Source: CAD feature listing. Evaluate the final solid. Frame: model axes, mm. Give positions to 0.01 mm unless a question says otherwise; leave off trailing zeros. Use a Markdown table: item, result. Add a question column.
```python
from build123d import *

# Parameters (mm, degrees)
SKETCH1_R           = 1.75
BOSS_EXTRUDE1_DEPTH = 5
CUT_EXTRUDE1_DEPTH  = 5
FILLET2_R           = 2


with BuildPart() as part:
    # Sketch1 → Boss-Extrude1 (new body)
    with BuildSketch(Plane(origin=(0, 0, 0), x_dir=(1, 0, 0), z_dir=(0, 1, 0))):
        with BuildLine():
            Line((-115, 97), (-115, -97))
            ThreePointArc((-115, -97), (-114.121320344, -99.121320344), (-112, -100))
            Line((-112, -100), (112, -100))
            ThreePointArc((112, -100), (114.121320344, -99.121320344), (115, -97))
            Line((115, -97), (115, 8.326847539))
            ThreePointArc((115, 8.326847539), (114.595001354, 9.832160786), (113.489354684, 10.931040816))
            Line((113.489354684, 10.931040816), (112.482257806, 11.50700592))
            Line((112.482257806, 11.50700592), (-41.694544071, 99.604753313))
            ThreePointArc((-41.694544071, 99.604753313), (-42.412938544, 99.899505125), (-43.182919083, 100))
            Line((-43.182919083, 100), (-112, 100))
            ThreePointArc((-112, 100), (-114.121320344, 99.121320344), (-115, 97))
        make_face()
        with Locations(Location((-107.357965586, 91.996726093, 0), (0, 0, 270))):
            Circle(SKETCH1_R, mode=Mode.SUBTRACT)
        with Locations(Location((107.171572875, 4.338256462, 0), (0, 0, 270))):
            Circle(SKETCH1_R, mode=Mode.SUBTRACT)
        with Locations(Location((107.171572875, -92.171572875, 0), (0, 0, 270))):
            Circle(SKETCH1_R, mode=Mode.SUBTRACT)
        with Locations(Location((-107.320588757, -92.030024345, 0), (0, 0, 270))):
            Circle(SKETCH1_R, mode=Mode.SUBTRACT)
    extrude(amount=BOSS_EXTRUDE1_DEPTH)

    # Sketch2 → Cut-Extrude1 (cut)
    with BuildSketch(Plane(origin=(0, 5, 0), x_dir=(1, 0, 0), z_dir=(0, 1, 0))):
        with BuildLine():
            ThreePointArc((83.411536631, -17.554766753), (65, -11.836576231), (46.588463369, -17.554766753))
            Line((46.588463369, -17.554766753), (83.411536631, -17.554766753))
        make_face()
        with BuildLine():
            ThreePointArc((42.258724115, -21.118385708), (39.509391878, -24.17525441), (37.167988383, -27.554766753))
            Line((37.167988383, -27.554766753), (92.832011617, -27.554766753))
            ThreePointArc((92.832011617, -27.554766753), (90.490608122, -24.17525441), (87.741275885, -21.118385708))
            Line((87.741275885, -21.118385708), (42.258724115, -21.118385708))
        make_face()
        with BuildLine():
            Line((94.690561452, -31.118385708), (35.309438548, -31.118385708))
            ThreePointArc((35.309438548, -31.118385708), (34.094437197, -34.281916226), (33.215458786, -37.554766753))
            Line((33.215458786, -37.554766753), (96.784541214, -37.554766753))
            ThreePointArc((96.784541214, -37.554766753), (95.905562803, -34.281916226), (94.690561452, -31.118385708))
        make_face()
        with BuildLine():
            Line((97.340272877, -41.118385708), (32.659727123, -41.118385708))
            ThreePointArc((32.659727123, -41.118385708), (32.5, -44.336576231), (32.659727123, -47.554766753))
            Line((32.659727123, -47.554766753), (97.340272877, -47.554766753))
            ThreePointArc((97.340272877, -47.554766753), (97.460043658, -45.94765219), (97.5, -44.336576231))
            ThreePointArc((97.5, -44.336576231), (97.460043658, -42.725500271), (97.340272877, -41.118385708))
        make_face()
        with BuildLine():
            Line((96.784541214, -51.118385708), (33.215458786, -51.118385708))
            ThreePointArc((33.215458786, -51.118385708), (34.094437197, -54.391236236), (35.309438548, -57.554766753))
            Line((35.309438548, -57.554766753), (94.690561452, -57.554766753))
            ThreePointArc((94.690561452, -57.554766753), (95.905562803, -54.391236236), (96.784541214, -51.118385708))
        make_face()
        with BuildLine():
            Line((92.832011617, -61.118385708), (37.167988383, -61.118385708))
            ThreePointArc((37.167988383, -61.118385708), (39.509391878, -64.497898052), (42.258724115, -67.554766753))
            Line((42.258724115, -67.554766753), (87.741275885, -67.554766753))
            ThreePointArc((87.741275885, -67.554766753), (90.490608122, -64.497898052), (92.832011617, -61.118385708))
        make_face()
        with BuildLine():
            Line((83.411536631, -71.118385708), (46.588463369, -71.118385708))
            ThreePointArc((46.588463369, -71.118385708), (65, -76.836576231), (83.411536631, -71.118385708))
        make_face()
    extrude(amount=-CUT_EXTRUDE1_DEPTH, mode=Mode.SUBTRACT)

    # Fillet2
    fillet2_edges = [part.edges().sort_by_distance(p)[0] for p in [
        (-114.121320344, 5, 99.121320344),
        (0, 5, 100),
        (114.121320344, 5, 99.121320344),
        (115, 5, 44.336576231),
        (114.595001354, 5, -9.832160786),
        (112.985806245, 5, -11.219023368),
        (35.393856868, 5, -55.555879616),
        (-42.412938544, 5, -99.899505125),
        (-77.591459542, 5, -100),
        (-114.121320344, 5, -99.121320344),
        (-115, 5, 0),
    ]]
    fillet(fillet2_edges, radius=FILLET2_R)


solid = part.part
```
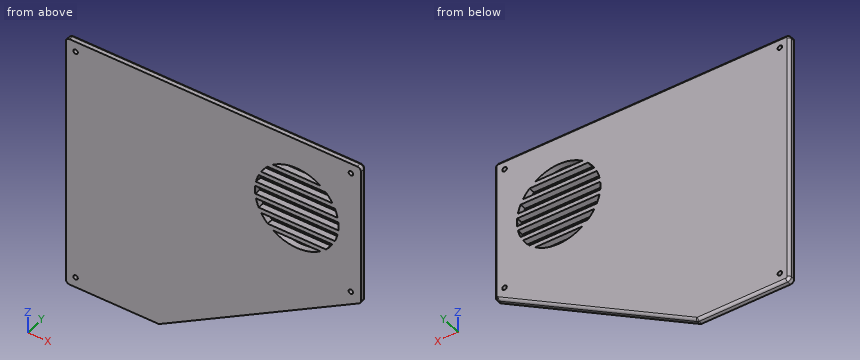
(1) First-contact query: pin 1 Ø1.5 at (x, y) = (59, 1.5) entering from -Z; pin 2 Ø1.5 at (x, y) = (67.5, 3) entering from -Z; pin 3 Ø3 at (x, z) = (107.17, 92.17) entering from -Y; pin 4 Ø3 at (x, y) = (41.5, 0.5) entering from -Z. Flat tips, straight axial feed; report the tip coordinate or a pass-through.
(2) Material intervals for L1, parallel to X at y = 2.25, z = 44.5; L2, parallel to X at y = 3.3, z = 2; L3, parallel to X at y = 2.1, z = 16, sorted ascending.
(3) Cut plane A-A on y = 1.6. Count the separate pieces of the cut face and the enclosed holes in it, then the cut area to 3 significant figures.
Output:
| question | item | result |
|---|---|---|
| 1 | pin 1 | z = -42.5 |
| 1 | pin 2 | z = -37.64 |
| 1 | pin 3 | through |
| 1 | pin 4 | z = -52.92 |
| 2 | L1 | -115 to 32.5, 97.5 to 115 |
| 2 | L2 | -114.98 to 114.98 |
| 2 | L3 | -115 to 49.08, 80.92 to 115 |
| 3 | separate pieces | 1 |
| 3 | enclosed holes | 11 |
| 3 | area | 36,700 mm^2 |
